from build123d import *

# Parameters (mm, degrees)
SKETCH1_W                = 13
SKETCH1_H                = 19
BOSS_EXTRUDE1_DEPTH      = 14.5
SKETCH2_W                = 15
SKETCH2_H                = 21
BOSS_EXTRUDE2_DEPTH      = 2
BOSS_EXTRUDE3_DEPTH      = 5.5
BOSS_EXTRUDE3_DEPTH_BACK = 5.5


with BuildPart() as part:
    # Sketch1 → Boss-Extrude1 (new body)
    with BuildSketch(Plane.XY):
        Rectangle(SKETCH1_W, SKETCH1_H)
    extrude(amount=BOSS_EXTRUDE1_DEPTH)

    # Sketch2 → Boss-Extrude2 (add)
    with BuildSketch(Plane.XY):
        Rectangle(SKETCH2_W, SKETCH2_H)
    extrude(amount=-BOSS_EXTRUDE2_DEPTH)

    # Sketch3 → Boss-Extrude3 (add, two sides: drawn at the far end of the back side and taken through both)
    with BuildSketch(Plane(origin=(0, 0, 0), x_dir=(0, 0, -1), z_dir=(1, 0, 0)).offset(-BOSS_EXTRUDE3_DEPTH_BACK)):
        with BuildLine():
            Line((2, -7.5), (2, 6))
            add(Edge.make_bspline(
                [(5.5, 4), (4.114672483, 5.598162681), (2, 6)],
                knots=[0, 0, 0, 1, 1, 1], degree=2))
            add(Edge.make_bspline(
                [(2, -7.5), (3.536685503, 1.127808031), (5.5, 4)],
                knots=[0, 0, 0, 1, 1, 1], degree=2))
        make_face()
    extrude(amount=BOSS_EXTRUDE3_DEPTH + BOSS_EXTRUDE3_DEPTH_BACK)


solid = part.part
Input: part model. Units: mm. Frame: model coordinates. A direction names the side the tool comes from. Give positions to 0.01 mm unless a question says otherwise; leave off trailing zeros. Loops run counter-clockwise (first coordinate to the right, second up) from the corner with the lowest first, then second, coordinate; pieces in that order, holes last. Notation, with made-up numbers: (28, -12.5) -> (79, -12.5) arc R16 cw to (79, 1.5) -> close; hole circle Ø2 at (64.25, -34.75). An arc over 180 degrees is marked (long way). Answer as a JSON object with one key per item and string values. Group by question number.
Item 1: Pull-direction query (Z, two-part tool) for faces 4 (the flat face through (0, 7, -2)), 5 (the flat face through (0, 0, 14.5)), 6 (the flat face through (-5.5, 2, -3)); classes: released by +Z, released by -Z, zero draft, split by the parting line, or undercut.
Item 2: Reachability of faces 1 (the flat face through (0, -9.5, 7)), 2 (the flat face through (0, 9.5, 7)), 3 (the flat face through (6.5, 0, 7)) from +Z, -Z, +X, -X, +Y, -Y: full face, straight path, thin tool, end or side. Return the list, or none.
Item 3: Pin query (flat end, axial travel): P1, Ø8, axis at y = -7.5, z = 10.5, coming from the +X side; P2, Ø8, axis at x = 2, z = 8, coming from the +Y side; P3, Ø10, axis at y = 4, z = 8, coming from the -X side; P4, Ø1.1, axis at y = -3, z = -4, coming from the -X side. Return the tip coordinate at first contact, or that it passes through.
Item 4: Cut plane A-A, the plane y = -8. Return the cut outline in (x, z), and give its area (4 significant figures).
Item 5: Line query: probe 1 along X at (y, z) = (3.25, -2.5); probe 2 along Z at (x, y) = (5.75, -5.75); probe 3 along X at (y, z) = (5, 10.5). Output: solid intervals per line, ascending.
Item 6: Cut plane B-B, the plane z = 6.5. Return the cut outline in (x, y), and give its area (3 significant figures).
Checks:
{
 "1": {"face 4": "released by -Z", "face 5": "released by +Z", "face 6": "zero draft"},
 "2": {"face 1": "+Z, +X, -X, -Y", "face 2": "+Z, +X, -X, +Y", "face 3": "+Z, +X, +Y, -Y"},
 "3": {"P1": "stops at x = 6.5", "P2": "stops at y = 9.5", "P3": "stops at x = -6.5", "P4": "passes through"},
 "4": {"outline": "(-7.5, -2) -> (7.5, -2) -> (7.5, 0) -> (6.5, 0) -> (6.5, 14.5) -> (-6.5, 14.5) -> (-6.5, 0) -> (-7.5, 0) -> close", "area": "218.5 mm²"},
 "5": {"probe 1": "x = -5.5 to 5.5", "probe 2": "z = -2 to 14.5", "probe 3": "x = -6.5 to 6.5"},
 "6": {"outline": "(-6.5, -9.5) -> (6.5, -9.5) -> (6.5, 9.5) -> (-6.5, 9.5) -> close", "area": "247 mm²"}
}
